Autodesk Inventor part; units mm, degrees
ref_plane "YZ Plane" through (0, 0, 0) normal (1, 0, 0) x (0, 1, 0)
ref_plane "XZ Plane" through (0, 0, 0) normal (0, 1, 0) x (-1, 0, 0)
ref_plane "XY Plane" through (0, 0, 0) normal (0, 0, 1) x (1, 0, 0)
sketch "Sketch1" plane through (0, 0, 0) normal (0, 1, 0) x (-1, 0, 0)
  circle A0 centre (0, 0) radius 5
  circle A1 centre (0, 0) radius 3
  dimension "d35" = 10
  dimension "d36" = 6
extrude "Extrusion11" add sketch "Sketch1" along normal blind 4 contours A1
extrude "Extrusion12" add sketch "Sketch1" along normal blind 1
draft "FaceDraft2" angle 33.5 pull direction (0, 1, 0) faces at (-2.9903, 3, -0.2414) fixed edges at (3, 4, 0)
sketch "Sketch8" plane through (0, 4, 0) normal (0, 1, 0) x (1, 0, 0)
  circle A0 centre (0, 0) radius 3.5
  dimension "d42" = 7
extrude "Extrusion13" add sketch "Sketch8" along normal blind 5
chamfer "Chamfer2" distance 0.5 angle 45 1 edges at (-3.5, 4, 0)
fillet "Fillet1" radius 1 1 edges at (-3.5, 4.4999, 0)
sketch "Sketch9" plane through (0, 9, 0) normal (0, 1, 0) x (1, 0, 0)
  circle A0 centre (0, 0) radius 4
  line L0 (3.5, -1.9365) -> (0.0729, -3.9993)
  line L1 (0.0729, -3.9993) -> (-3.4271, -2.0628)
  line L2 (-3.4271, -2.0628) -> (-3.5, 1.9365)
  line L3 (-3.5, 1.9365) -> (-0.0729, 3.9993)
  line L4 (-0.0729, 3.9993) -> (3.4271, 2.0628)
  line L5 (3.4271, 2.0628) -> (3.5, -1.9365)
  circle A1 centre (0, 0) radius 3.5
  point P0 (1.3581, -3.2258)
  point P1 (-1.2396, -3.2732)
  point P2 (-2.1146, -2.789)
  point P3 (-3.4544, -0.5631)
  point P4 (-3.4726, 0.4367)
  point P5 (-2.2149, 2.7101)
  point P6 (-1.3581, 3.2258)
  point P7 (1.2396, 3.2732)
  point P8 (2.1146, 2.789)
  point P9 (3.4544, 0.5631)
  point P10 (3.4726, -0.4367)
  point P11 (2.2149, -2.7101)
  dimension "d49" = 8
extrude "Extrusion14" add sketch "Sketch9" along normal blind 7 contours L5 A1 L4 | L0 A1 L5 | L4 A1 L3 | A1 L5 L0 L1 L2 L3 L4 | L1 A1 L0 | L3 A1 L2 | L2 A1 L1
sketch "Sketch10" plane through (0, 16, 0) normal (0, 1, 0) x (1, 0, 0)
  circle A0 centre (0, 0) radius 2.5
  circle A1 centre (0, 0) radius 2.25
  dimension "d54" = 5
  dimension "d55" = 4.5
extrude "Extrusion16" add sketch "Sketch10" along normal blind 0.5 contours A1
sketch "Sketch11" plane through (0, 16.5, 0) normal (0, 1, 0) x (1, 0, 0)
  circle A0 centre (0, 0) radius 2.5
  dimension "d58" = 5
extrude "Extrusion18" add sketch "Sketch11" along normal blind 5
fillet "Fillet2" radius 0.5 1 edges at (-2.25, 16.5, 0)
thread "Thread2"
chamfer "Chamfer3" distance 0.5 angle 45 1 edges at (-2.5, 21.5, 0)
sketch "Sketch12" plane through (0, 0, 0) normal (0, -1, 0) x (1, 0, 0)
  circle A0 centre (0, 0) radius 4
  dimension "d70" = 8
extrude "Extrusion19" cut sketch "Sketch12" against normal blind 2
fillet "Fillet3" radius 0.5 1 edges at (-4, 2, 0)
sketch "Sketch13" plane through (0, 21.5, 0) normal (0, 1, 0) x (1, 0, 0)
  circle A0 centre (0, 0) radius 1
  dimension "d74" = 2
extrude "Extrusion20" cut sketch "Sketch13" against normal up to next
properties part number "cup"
Geometry check sheet. Reference: the model listing, model coordinates, mm. A direction names the side the tool comes from. Give positions to 0.01 mm unless a question says otherwise; leave off trailing zeros. Loops run counter-clockwise (first coordinate to the right, second up) from the corner with the lowest first, then second, coordinate; pieces in that order, holes last.
(1) Depth check by flat-ended pin: pin 1 Ø1 at (x, z) = (-1, 3) entering from -Y; pin 2 Ø3 at (x, y) = (-3.5, 7) entering from +Z; pin 3 Ø3 at (x, y) = (3.5, 11) entering from +Z. Enter the tip coordinate at first touch or a pass-through.
From the geometry:
pin 1: stops at y = 1.97
pin 2: stops at z = 2.87
pin 3: stops at z = 2.84
(2) Thickness scan on L1, parallel to Z at x = 0, y = 0.45; L2, parallel to Y at x = -0.75, z = -1; L3, parallel to Z at x = 0, y = 15.75. Record the ranges inside material, lowest first.
From the geometry:
L1: z = -5 to -4, 4 to 5
L2: y = 2 to 21.5
L3: z = -3.96 to -1, 1 to 3.96
(3) Section check B-B on y = 18.75. Record the cut outline in (x, z).
From the geometry:
outline: circle Ø5 at (0, 0); hole circle Ø2 at (0, 0)
(4) Section check C-C on y = 6.25. Record the cut outline in (x, z), then the cut area to 3 significant figures.
From the geometry:
outline: circle Ø7 at (0, 0); hole circle Ø2 at (0, 0)
area: 35.3 mm2
(5) Section check A-A on y = 15. Record the cut outline in (x, z), then the cut area to 3 significant figures.
From the geometry:
outline: (-3.5, -1.94) - (-0.07, -4) - (3.43, -2.06) - (3.5, 1.94) - (0.07, 4) - (-3.43, 2.06) - close; hole circle Ø2 at (0, 0)
area: 38.4 mm2
(6) Release check for a two-part mould opening along Z. For faces 5 (the cylindrical face through (0, 12, 1)), 6 (the flat face through (-3.14, 9, 1.92)), 7 (the flat face through (1.81, 12.451, 2.953)) record: released by +Z, released by -Z, zero draft, split by the parting line, or undercut.
From the geometry:
face 5: undercut
face 6: zero draft
face 7: released by +Z
(7) Set-up check for faces 1 (the flat face through (-3.24, 9, -1.75)), 2 (the flat face through (3.2, 9, -1.8)), 3 (the cylindrical face through (-0.54, 18.72, -2.44)), 4 (the flat face through (1, 2, -1)): record each of +Z, -Z, +X, -X, +Y, -Y from which the full face is reachable in a straight line by a thin tool's end or side.
From the geometry:
face 1: -Z, -X
face 2: -Z, +X
face 3: +Y
face 4: -Y
